from build123d import *

# Parameters (mm, degrees)
BOSS_EXTRUDE1_DEPTH = 150
SKETCH4_R           = 1.65
CUT_EXTRUDE1_DEPTH  = 10
SKETCH6_W           = 1.5
SKETCH6_H           = 150
CUT_EXTRUDE2_DEPTH  = 2
SKETCH7_R           = 2.5
CUT_EXTRUDE3_DEPTH  = 7


with BuildPart() as part:
    # Sketch1 → Boss-Extrude1 (new body)
    with BuildSketch(Plane.XY):
        Polygon((-75.5, 5), (75.5, 5), (75.5, -5), (23.151457837, -5), (23.151457837, -15), (17.151457837, -15), (17.151457837, -5), (-17.151457837, -5), (-17.151457837, -15), (-23.151457837, -15), (-23.151457837, -5), (-75.5, -5), align=None)
    extrude(amount=BOSS_EXTRUDE1_DEPTH)

    # Sketch4 → Cut-Extrude1 (cut)
    with BuildSketch(Plane.XZ.offset(5)):
        with Locations((-10, 6)):
            Circle(SKETCH4_R)
        with Locations((10, 6)):
            Circle(SKETCH4_R)
        with Locations((-10, 144)):
            Circle(SKETCH4_R)
        with Locations((10, 144)):
            Circle(SKETCH4_R)
    extrude(amount=-CUT_EXTRUDE1_DEPTH, mode=Mode.SUBTRACT)

    # Sketch6 → Cut-Extrude2 (cut)
    with BuildSketch(Plane(origin=(0, 5, 0), x_dir=(1, 0, 0), z_dir=(0, 1, 0))):
        with Locations((-24.75, -75)):
            Rectangle(SKETCH6_W, SKETCH6_H)
        with Locations((24.75, -75)):
            Rectangle(SKETCH6_W, SKETCH6_H)
    extrude(amount=-CUT_EXTRUDE2_DEPTH, mode=Mode.SUBTRACT)

    # Sketch7 → Cut-Extrude3 (cut)
    with BuildSketch(Plane(origin=(0, 5, 0), x_dir=(1, 0, 0), z_dir=(0, 1, 0))):
        with Locations((-10, -144)):
            Circle(SKETCH7_R)
        with Locations((10, -144)):
            Circle(SKETCH7_R)
        with Locations((10, -6)):
            Circle(SKETCH7_R)
        with Locations((-10, -6)):
            Circle(SKETCH7_R)
    extrude(amount=-CUT_EXTRUDE3_DEPTH, mode=Mode.SUBTRACT)


solid = part.part
The listing builds one solid part. Answer for the finished solid, in the listing's coordinates (mm). A direction names the side the tool comes from. Coordinates: 2 decimals unless noted, no trailing zeros. Loops run counter-clockwise (first coordinate to the right, second up) from the corner with the lowest first, then second, coordinate; pieces in that order, holes last. Notation, with made-up numbers: (21, 17) -> (56, 17) arc R23 ccw to (56, 52) -> close; hole circle Ø1 at (17, 40). An arc over 180 degrees is marked (long way). Answer in a Markdown table with one row per item. Add a question column.
1. Determine the mould class of faces 5 (the flat face through (-9, -2, 8)), 6 (the flat face through (-20, -15, 74)), 7 (the flat face through (1, 0, 0)) for opening direction Z: +Z half, -Z half, draft (parallel to the pull), parting line (faces both ways), or undercut.
2. Flat-ended cylindrical pins translate along their axes: P1, Ø4.5, axis at x = 10, z = 144, coming from the -Y side; P2, Ø5, axis at y = -8, z = 68.5, coming from the -X side; P3, Ø5, axis at y = -12.5, z = 67, coming from the +X side. Find the tip coordinate at first contact, or state that the pin passes through.
3. The part is cut by section A-A, the plane y = -11.5. Write down the section's boundary in (x, z), then the cut area to 3 significant figures.
4. Consider line 1 (Z direction, x = -10, y = 0.5); line 2 (X direction, y = 3.5, z = 6); line 3 (Z direction, x = -10, y = -2.8). Determine where each line is inside the solid, lowest interval first. Write a range as [from, to].
5. The part is cut by section B-B, the plane z = 103.5. Write down the section's boundary in (x, y).
6. The part is cut by section C-C, the plane x = -31. Write down the section's boundary in (y, z), then the cut area to 3 significant figures.
7. For faces 1 (the flat face through (23.151, -10, 74)), 2 (the flat face through (17.151, -10, 74)), 3 (the cylindrical face through (8.16, 1.55, 4.31)), 4 (the flat face through (-23.151, -10, 74)), determine the directions among +Z, -Z, +X, -X, +Y, -Y from which every point of the face is accessible in a straight line to the end or side of a thin tool.
Answer below:
| question | item | result |
|---|---|---|
| 1 | face 5 | undercut |
| 1 | face 6 | draft |
| 1 | face 7 | -Z half |
| 2 | P1 | y = -5 |
| 2 | P2 | x = -23.15 |
| 2 | P3 | x = 23.15 |
| 3 | outline | (-23.15, 0) -> (-17.15, 0) -> (-17.15, 150) -> (-23.15, 150) -> close; (17.15, 0) -> (23.15, 0) -> (23.15, 150) -> (17.15, 150) -> close |
| 3 | area | 1,800 mm2 |
| 4 | line 1 | [0, 3.5], [8.5, 141.5], [146.5, 150] |
| 4 | line 2 | [-75.5, -25.5], [-24, -12.5], [-7.5, 7.5], [12.5, 24], [25.5, 75.5] |
| 4 | line 3 | [0, 4.35], [7.65, 142.35], [145.65, 150] |
| 5 | outline | (-75.5, -5) -> (-23.15, -5) -> (-23.15, -15) -> (-17.15, -15) -> (-17.15, -5) -> (17.15, -5) -> (17.15, -15) -> (23.15, -15) -> (23.15, -5) -> (75.5, -5) -> (75.5, 5) -> (25.5, 5) -> (25.5, 3) -> (24, 3) -> (24, 5) -> (-24, 5) -> (-24, 3) -> (-25.5, 3) -> (-25.5, 5) -> (-75.5, 5) -> close |
| 6 | outline | (-5, 0) -> (5, 0) -> (5, 150) -> (-5, 150) -> close |
| 6 | area | 1,500 mm2 |
| 7 | face 1 | +Z, -Z, +X, -Y |
| 7 | face 2 | +Z, -Z, -Y |
| 7 | face 3 | +Y |
| 7 | face 4 | +Z, -Z, -X, -Y |
